The model under review builds one solid part; all positions refer to its coordinate system, in mm. Face numbers are marked on the shaded views. A direction names the side the tool comes from. Round coordinates to 2 decimals unless told otherwise and drop trailing zeros. Write each loop counter-clockwise with the first axis right and the second up, starting at its lowest first coordinate (ties: lowest second). Pieces come first, ordered by that corner, then holes.
Item 1: Add section A-A (z = 52). Give the boundary of the cut face in (x, y).
Item 2: Machinability: for the marked faces 1 and 2, which of the approach directions +Z, -Z, +X, -X, +Y, -Y give a long, thin tool a straight path to every point of the face, cutting with its end or side? Answer none if there is none.
Item 3: Clearance check with flat-ended pins moving along their axes: pin 1 Ø12 at (y, z) = (48, 25.5) entering from +X; pin 2 Ø3 at (x, z) = (-30, 19) entering from +Y; pin 3 Ø6 at (x, z) = (27.5, 8.5) entering from +Y; pin 4 Ø10 at (x, y) = (8, 88) entering from -Z. State where each tip first meets the part, or that it passes through.
Item 4: Add section C-C (x = -12.5). Give the boundary of the cut face in (y, z), plus the area to 3 significant figures.
Item 5: To check wall thickness, follow L1, parallel to X at y = 77, z = 47.5; L2, parallel to Y at x = -3, z = 34; L3, parallel to X at y = 104.5, z = 10. State the ranges of each line that lie inside material, in increasing order.
Item 6: Add section B-B (y = 83). Give the boundary of the cut face in (x, z).
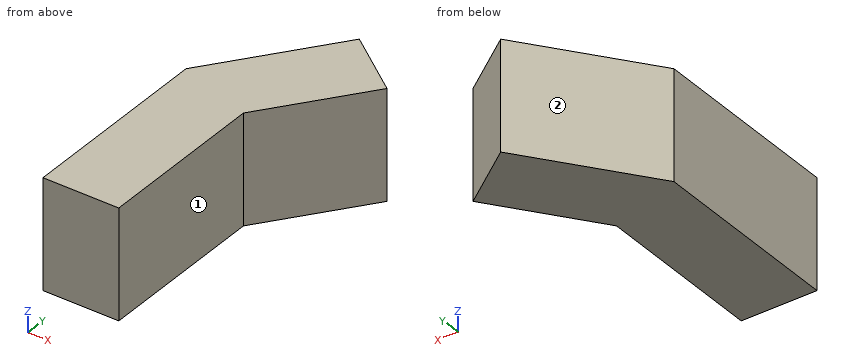
```python
from build123d import *

# Parameters (mm, degrees)
F0_W = 40.0777868927
F0_H = 57.9875484109


with BuildPart() as f2:
    # F2: sweep along a path in F1
    with BuildLine(Plane.XY) as f2_path:
        Line((-40.0777868927, 0), (-40.0777868927, 104.355700314))
        Line((-40.0777868927, 104.355700314), (6.5287379548, 166.5153428912))
    # F0 (on Front) → F2 (sweep)
    with BuildSketch(Plane.XZ):
        with Locations((-20.0388934463, 28.9937742054)):
            Rectangle(F0_W, F0_H)
    sweep(path=f2_path.line, transition=Transition.RIGHT)


solid = f2.part
```
Numbers:
1. outline: (-40.08, 0) - (0, 0) - (0, 91) - (38.59, 142.47) - (6.53, 166.52) - (-40.08, 104.36) - close
2. face 1: +Z, -Z, +X, -Y
2. face 2: +Z, -Z, -X, +Y
3. pin 1: stops at x = 0
3. pin 2: stops at y = 119.8
3. pin 3: stops at y = 153.04
3. pin 4: passes through
4. outline: (0, 0) - (141.14, 0) - (141.14, 57.99) - (0, 57.99) - close
4. area: 8,180 mm2
5. L1: x = -40.08 to 0
5. L2: y = 0 to 153.81
5. L3: x = -39.97 to 10.12
6. outline: (-40.08, 0) - (0, 0) - (0, 57.99) - (-40.08, 57.99) - close
